Autodesk Inventor part; units mm, degrees
ref_plane "YZ Plane" through (0, 0, 0) normal (1, 0, 0) x (0, 1, 0)
ref_plane "XZ Plane" through (0, 0, 0) normal (0, 1, 0) x (-1, 0, 0)
ref_plane "XY Plane" through (0, 0, 0) normal (0, 0, 1) x (1, 0, 0)
sketch "Esquisse1" plane through (0, 0, 0) normal (0, 1, 0) x (-1, 0, 0)
  line L0 (-15, 20) -> (15, 20)
  line L1 (15, 20) -> (15, -20)
  line L2 (15, -20) -> (-15, -20)
  line L3 (-15, -20) -> (-15, 20)
  line L4 (-15, 20) -> (15, -20) construction
  line L5 (15, 20) -> (-15, -20) construction
  point P0 (0, 0)
  dimension "d0" = 30
  dimension "d1" = 40
extrude "Extrusion1" add sketch "Esquisse1" along normal blind 2
sketch "Esquisse2" plane through (0, 2, 0) normal (0, 1, 0) x (1, 0, 0)
  line L0 (10, -10) -> (-10, -10)
  line L1 (-10, -10) -> (-10, 10)
  line L2 (-10, 10) -> (10, 10)
  line L3 (10, 10) -> (10, -10)
  line L4 (10, -10) -> (-10, 10) construction
  line L5 (-10, -10) -> (10, 10) construction
  point P0 (0, 0)
  dimension "d4" = 20
  dimension "d5" = 20
extrude "Extrusion2" add sketch "Esquisse2" along normal blind 66
sketch "Esquisse3" plane through (0, 68, 0) normal (0, 1, 0) x (1, 0, 0)
  line L0 (7.5, 7.5) -> (-7.5, 7.5)
  line L1 (-7.5, 7.5) -> (-7.5, -7.5)
  line L2 (-7.5, -7.5) -> (7.5, -7.5)
  line L3 (7.5, -7.5) -> (7.5, 7.5)
  line L4 (7.5, 7.5) -> (-7.5, -7.5) construction
  line L5 (-7.5, 7.5) -> (7.5, -7.5) construction
  point P0 (0, 0)
  dimension "d9" = 15
  dimension "d10" = 15
extrude "Extrusion3" cut sketch "Esquisse3" against normal through all
sketch "Esquisse4" plane through (0, 2, 0) normal (0, 1, 0) x (1, 0, 0)
  line L0 (0, 0) -> (0, -15)
  line L1 (0, -15) -> (-7.5, -15)
  line L2 (0, 0) -> (0, 15)
  line L3 (0, 15) -> (-7.5, 15)
  point P0 (7.5, -15)
  point P1 (7.5, 15)
  point P2 (7.5, 15)
  dimension "d13" = 15
  dimension "d14" = 7.5
  dimension "d15" = 15
  dimension "d16" = 7.5
hole "Perçage1" at (-7.5, 2, 15) at (7.5, 2, 15) at (-7.5, 2, -15) at (7.5, 2, -15) direction (0, -1, 0) diameter 2.459 end through all
sketch "Esquisse5" plane through (10, 2, -10) normal (0, 0, -1) x (-1, 0, 0)
  point P0 (10, -2)
sketch "Esquisse6" plane through (10, 2, -10) normal (0, 0, -1) x (-1, 0, 0)
  line L0 (0, 66) -> (20, 66)
  line L1 (0, 66) -> (0, 61)
  line L2 (0, 0) -> (0, 66)
  line L3 (20, 0) -> (20, 66)
  line L4 (0, 61) -> (20, 61)
  line L5 (20, 61) -> (20, 58)
  line L6 (20, 58) -> (0, 58)
  line L7 (0, 58) -> (0, 61)
  point P0 (10, -2)
  point P1 (0, 58)
  dimension "d24" = 5
  dimension "d25" = 3
extrude "Extrusion4" add sketch "Esquisse6" along normal blind 5 contours L4 L3 L6 L2
sketch "Esquisse7" plane through (-10, 2, 10) normal (0, 0, 1) x (1, 0, 0)
  line L0 (0, 66) -> (20, 66)
  line L1 (0, 66) -> (0, 61)
  line L2 (0, 0) -> (0, 66)
  line L3 (20, 0) -> (20, 58)
  line L4 (0, 61) -> (20, 61)
  line L5 (20, 61) -> (20, 58)
  line L6 (20, 58) -> (0, 58)
  line L7 (0, 58) -> (0, 61)
  point P0 (10, -2)
  point P1 (0, 58)
  dimension "d28" = 5
  dimension "d29" = 3
extrude "Extrusion5" add sketch "Esquisse7" along normal blind 5
sketch "Esquisse8" plane through (10, 2, 10) normal (1, 0, 0) x (0, 0, -1)
  line L0 (-5, 61) -> (-5, 58)
  line L1 (20, 58) -> (25, 58)
  line L2 (-5, 61) -> (25, 61)
  line L3 (25, 61) -> (25, 58)
  line L4 (25, 58) -> (-5, 58)
  line L5 (-5, 58) -> (-5, 61)
  point P0 (10, -2)
extrude "Extrusion6" add sketch "Esquisse8" along normal blind 5
sketch "Esquisse9" plane through (-10, 2, -10) normal (-1, 0, 0) x (0, 0, 1)
  line L0 (-5, 58) -> (-5, 61)
  line L1 (25, 61) -> (25, 58)
  line L2 (-5, 61) -> (25, 61)
  line L3 (25, 61) -> (25, 58)
  line L4 (25, 58) -> (-5, 58)
  line L5 (-5, 58) -> (-5, 61)
  point P0 (10, -2)
extrude "Extrusion7" add sketch "Esquisse9" along normal blind 5
fillet "Congé2" radius 2 8 edges at (10, 31, -10) (10, 31, 10) (10, 2, 0) (0, 2, -10) (-10, 31, -10) (-10, 2, 0) (-10, 31, 10) (0, 2, 10)
fillet "Congé3" radius 2 8 edges at (-9.4142, 60, -9.4142) (0, 60, -10) (9.4142, 60, -9.4142) (10, 60, 0) (9.4142, 60, 9.4142) (0, 60, 10) (-9.4142, 60, 9.4142) (-10, 60, 0)
properties part number "Bras caméra"
Can you work these out from the model? Positions are in its coordinate system, mm. A direction names the side the tool comes from. Round coordinates to 2 decimals unless told otherwise and drop trailing zeros. Order: outer loops, then holes, each group sorted by start corner. A loop starts at its lowest first (then second) coordinate and runs counter-clockwise, first axis right, second up. Notation, with made-up numbers: M 55,1 L 99,1 A26 cw 99,19 Z; hole C -5,71 d1. An arc over 180 degrees is marked long. Use a Markdown table: item, result.
1) Imagine slicing it at A-A (x = -4). List the corners of the cut face in (y, z) for me, then the cut area to 3 significant figures.
Geometry says:
| item | result |
|---|---|
| outline | M 0,-20 L 2,-20 L 2,-12 A2 cw 4,-10 L 58,-10 A2 cw 60,-12 L 60,-15 L 63,-15 L 63,-10 L 68,-10 L 68,-7.5 L 0,-7.5 Z; M 0,7.5 L 68,7.5 L 68,10 L 63,10 L 63,15 L 60,15 L 60,12 A2 cw 58,10 L 4,10 A2 cw 2,12 L 2,20 L 0,20 Z |
| area | 413 mm² |
2) Imagine slicing it at D-D (y = 61.5). List the corners of the cut face in (x, z) for me.
Geometry says:
| item | result |
|---|---|
| outline | M -15,-15 L 15,-15 L 15,15 L -15,15 Z; hole M -7.5,-7.5 L 7.5,-7.5 L 7.5,7.5 L -7.5,7.5 Z |
3) If we mould it in two halves opening along Z, with no side actions, what happens to faces 1 (the face through (0, 1, -20)), 2 (the face through (-7.029, 0.986, 16.136)), 3 (the face through (0, 65, 10)), 4 (the face through (-15, 62, 0))? For each: +Z half, -Z half, draft (parallel to the pull), parting line (faces both ways), or undercut.
Geometry says:
| item | result |
|---|---|
| face 1 | -Z half |
| face 2 | undercut |
| face 3 | +Z half |
| face 4 | draft |
4) On a 3-axis mill with a long thin cutter (end or side, diameter ignored), from which of +Z, -Z, +X, -X, +Y, -Y can I reach the whole of each face in a straight line? I mean faces 5 (the face through (-10, 65, 0)), 6 (the face through (0, 34, -7.5)), 7 (the face through (-0.11, 59.43, 10.6)), 8 (the face through (0, 60, 14)). Say none if no direction works.
Geometry says:
| item | result |
|---|---|
| face 5 | +Z, -Z, -X, +Y |
| face 6 | +Y, -Y |
| face 7 | +Z, +X, -X |
| face 8 | none |
5) I'm going to push flat-ended pins straight in: P1, Ø5, axis at y = 36, z = 11, coming from the -X side; P2, Ø2, axis at x = -7.5, z = -15, coming from the -Y side; P3, Ø1.5, axis at x = -3, y = 62, coming from the +Z side. Where does each tip first touch, or does it pass through?
Geometry says:
| item | result |
|---|---|
| P1 | stops at x = -9.94 |
| P2 | stops at y = 60 |
| P3 | stops at z = 15 |
6) If I drill on line 1 along X through (y, z) = (1, 15); line 2 along X through (y, z) = (12.5, 5.5); line 3 along Y through (x, z) = (-13.5, -5.5), over which ranges is the centre line in solid material (lowest first)?
Geometry says:
| item | result |
|---|---|
| line 1 | x = -15 to -8.73, -6.27 to 6.27, 8.73 to 15 |
| line 2 | x = -10 to -7.5, 7.5 to 10 |
| line 3 | y = 0 to 2, 60 to 63 |
7) Imagine slicing it at C-C (z = 4). List the corners of the cut face in (x, y) for me.
Geometry says:
| item | result |
|---|---|
| outline | M -15,0 L -7.5,0 L -7.5,68 L -10,68 L -10,63 L -15,63 L -15,60 L -12,60 A2 cw -10,58 L -10,4 A2 cw -12,2 L -15,2 Z; M 7.5,0 L 15,0 L 15,2 L 12,2 A2 cw 10,4 L 10,58 A2 cw 12,60 L 15,60 L 15,63 L 10,63 L 10,68 L 7.5,68 Z |
8) Imagine slicing it at B-B (y = 23.5). List the corners of the cut face in (x, z) for me, then the cut area to 3 significant figures.
Geometry says:
| item | result |
|---|---|
| outline | M -10,-8 A2 ccw -8,-10 L 8,-10 A2 ccw 10,-8 L 10,8 A2 ccw 8,10 L -8,10 A2 ccw -10,8 Z; hole M -7.5,-7.5 L 7.5,-7.5 L 7.5,7.5 L -7.5,7.5 Z |
| area | 172 mm² |
